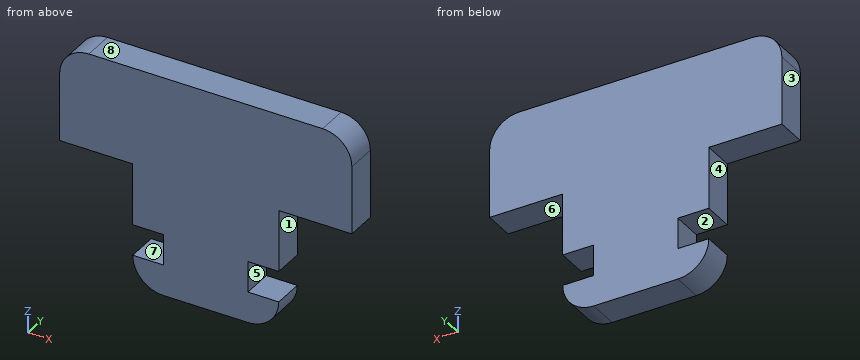
```python
from build123d import *

# Parameters (mm, degrees)
SKETCH1_W           = 30
SKETCH1_H           = 10
BOSS_EXTRUDE2_DEPTH = 3.175
FILLET3_R           = 3


with BuildPart() as part:
    # Sketch1 → Boss-Extrude2 (new body)
    with BuildSketch(Plane(origin=(0, 0, 0), x_dir=(1, 0, 0), z_dir=(0, 1, 0))):
        with Locations((0, -5)):
            Rectangle(SKETCH1_W, SKETCH1_H)
        Polygon((-7.5, 3.175), (-7.5, 0), (7.5, 0), (7.5, 3.175), (7.5, 6.35), (4.325, 6.35), (-3.85, 6.35), (-4.325, 6.35), (-7.5, 6.35), align=None)
        Polygon((-4.325, 9.525), (-4.325, 6.35), (-3.85, 6.35), (4.325, 6.35), (4.325, 9.525), align=None)
        with BuildLine():
            ThreePointArc((-7.5, 9.525), (-6.57006403, 11.77006403), (-4.325, 12.7))
            Line((-4.325, 12.7), (4.325, 12.7))
            ThreePointArc((4.325, 12.7), (6.57006403, 11.77006403), (7.5, 9.525))
            Line((7.5, 9.525), (4.325, 9.525))
            Line((4.325, 9.525), (-4.325, 9.525))
            Line((-4.325, 9.525), (-7.5, 9.525))
        make_face()
    extrude(amount=BOSS_EXTRUDE2_DEPTH)

    # Fillet3
    fillet3_edges = [part.edges().sort_by_distance(p)[0] for p in [
        (15, 1.5875, 10),
        (-15, 1.5875, 10),
    ]]
    fillet(fillet3_edges, radius=FILLET3_R)


solid = part.part
```
For this review, take the finished solid that the model builds, in its own axes (mm). Face numbers are marked on the shaded views. A direction names the side the tool comes from. Round coordinates to 2 decimals unless told otherwise and drop trailing zeros. Loops run counter-clockwise (first coordinate to the right, second up) from the corner with the lowest first, then second, coordinate; pieces in that order, holes last.
Q1. Insertion check: pin 1 Ø1.5 at (y, z) = (2, -2) entering from -X; pin 2 Ø1.5 at (x, z) = (10, -10) entering from -Y; pin 3 Ø1.6 at (y, z) = (1.5, -8.5) entering from +X (3 decimals); pin 4 Ø1 at (y, z) = (2, -3.5) entering from +X. Each pin has a flat end and moves straight along its axis. Give the tip position at first contact, or say it passes through.
Result sheet:
pin 1: stops at x = -7.5
pin 2: passes through
pin 3: stops at x = 4.325
pin 4: stops at x = 7.5
Q2. To check wall thickness, follow line 1 along Z through (x, y) = (-12, 1.6); line 2 along X through (y, z) = (2.95, -0.75); line 3 along Z through (x, y) = (-5.75, 1.7) (3 decimals). State the ranges of each line that lie inside material, in increasing order.
Result sheet:
line 1: z = 0 to 10
line 2: x = -7.5 to 7.5
line 3: z = -12.362 to -9.525, -6.35 to 10
Q3. Mouldability with a two-part tool opening along Z and no side actions: class the marked faces 6, 7 and 8 as +Z half, -Z half, draft (parallel to the pull), parting line (faces both ways), or undercut.
Result sheet:
face 6: -Z half
face 7: undercut
face 8: +Z half
Q4. Add section C-C on x = -8.75. Write out the cut boundary in (y, z) (3 decimals), plus the area to 4 significant figures.
Result sheet:
outline: (0, 0) - (3.175, 0) - (3.175, 10) - (0, 10) - close
area: 31.75 mm2
Q5. Add section A-A on y = 2.8. Write out the cut boundary in (x, z) (3 decimals).
Result sheet:
outline: (-15, 0) - (-7.5, 0) - (-7.5, -6.35) - (-4.325, -6.35) - (-4.325, -9.525) - (-7.5, -9.525) arc R3.175 ccw to (-4.325, -12.7) - (4.325, -12.7) arc R3.175 ccw to (7.5, -9.525) - (4.325, -9.525) - (4.325, -6.35) - (7.5, -6.35) - (7.5, 0) - (15, 0) - (15, 7) arc R3 ccw to (12, 10) - (-12, 10) arc R3 ccw to (-15, 7) - close
Q6. Machinability: for the marked faces 1, 2, 3, 4 and 5, which of the approach directions +Z, -Z, +X, -X, +Y, -Y give a long, thin tool a straight path to every point of the face, cutting with its end or side? Answer none if there is none.
Result sheet:
face 1: -Z, +X, +Y, -Y
face 2: -X, +Y, -Y
face 3: +Z, -Z, -X, +Y, -Y
face 4: -Z, -X, +Y, -Y
face 5: +X, +Y, -Y
Q7. Add section B-B on z = -4.25. Write out the cut boundary in (x, y) (3 decimals).
Result sheet:
outline: (-7.5, 0) - (7.5, 0) - (7.5, 3.175) - (-7.5, 3.175) - close
